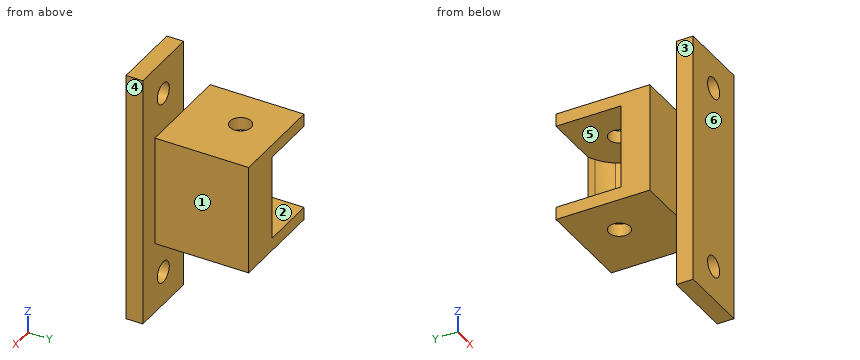
from build123d import *

# Parameters (mm, degrees)
BOSS_EXTRUDE1_DEPTH = 29.21
SKETCH2_R           = 3.175
BOSS_EXTRUDE2_DEPTH = 3.81
BOSS_EXTRUDE4_START = 3.81
SKETCH3_W           = 29.223613814
SKETCH3_H           = 28.25489527
SKETCH3_R           = 3.175
BOSS_EXTRUDE4_DEPTH = 3.81
SKETCH4_W           = 21.59
SKETCH4_H           = 76.2
SKETCH4_R           = 3.175
BOSS_EXTRUDE5_DEPTH = 5.08


with BuildPart() as part:
    # Sketch1 → Boss-Extrude1 (new body)
    with BuildSketch(Plane.XY):
        with BuildLine():
            Line((497.233946268, 332.485515977), (497.233946268, 323.779975182))
            Line((497.233946268, 323.779975182), (526.457560082, 323.779975182))
            Line((526.457560082, 323.779975182), (526.457560082, 352.034870452))
            Line((526.457560082, 352.034870452), (514.19218435, 352.034870452))
            Line((514.19218435, 352.034870452), (515.97416853, 351.010540676))
            ThreePointArc((515.97416853, 351.010540676), (518.254444166, 349.336379834), (520.107560082, 347.198990562))
            ThreePointArc((520.107560082, 347.198990562), (520.655570716, 333.67086151), (508.689794246, 327.335975182))
            ThreePointArc((508.689794246, 327.335975182), (505.910190066, 327.86159111), (503.31589155, 328.989459324))
            Line((503.31589155, 328.989459324), (497.233946268, 332.485515977))
        make_face()
    extrude(amount=-BOSS_EXTRUDE1_DEPTH)

    # Sketch2 → Boss-Extrude2 (add)
    with BuildSketch(Plane(origin=(0, 0, -25.4), x_dir=(-1, 0, 0), z_dir=(0, 0, -1))):
        with BuildLine():
            Line((-514.19218435, 352.034870452), (-497.233946268, 352.034870452))
            Line((-497.233946268, 352.034870452), (-497.233946268, 332.485515977))
            Line((-497.233946268, 332.485515977), (-503.31589155, 328.989459324))
            ThreePointArc((-503.31589155, 328.989459324), (-520.655570716, 333.67086151), (-515.97416853, 351.010540676))
            Line((-515.97416853, 351.010540676), (-514.19218435, 352.034870452))
        make_face()
        with Locations(Location((-509.64503004, 340, 0), (0, 0, 180))):
            Circle(SKETCH2_R, mode=Mode.SUBTRACT)
    extrude(amount=BOSS_EXTRUDE2_DEPTH)

    # Sketch3 → Boss-Extrude4 (add)
    with BuildSketch(Plane.XY.offset(BOSS_EXTRUDE4_START)):
        with Locations((511.845753175, 337.907422817)):
            Rectangle(SKETCH3_W, SKETCH3_H)
        with Locations((509.64503004, 340)):
            Circle(SKETCH3_R, mode=Mode.SUBTRACT)
    extrude(amount=-BOSS_EXTRUDE4_DEPTH)

    # Sketch4 → Boss-Extrude5 (add)
    with BuildSketch(Plane(origin=(0, 323.779975182, 0), x_dir=(1, 0, 0), z_dir=(0, 1, 0))):
        with Locations((522.012560082, 12.7)):
            Rectangle(SKETCH4_W, SKETCH4_H)
        with Locations(Location((522.012560082, 40.64, 0), (0, 0, 270))):
            Circle(SKETCH4_R, mode=Mode.SUBTRACT)
        with Locations(Location((522.012560082, -15.24, 0), (0, 0, 270))):
            Circle(SKETCH4_R, mode=Mode.SUBTRACT)
    extrude(amount=-BOSS_EXTRUDE5_DEPTH)


solid = part.part
Check sheet for the modelled part. Datum: model origin and axes. Units: mm. Face numbers are marked on the shaded views. A direction names the side the tool comes from. Round coordinates to 2 decimals unless told otherwise and drop trailing zeros. Order: outer loops, then holes, each group sorted by start corner. A loop starts at its lowest first (then second) coordinate and runs counter-clockwise, first axis right, second up.
(1) Cross-section at B-B, the plane y = 340. Enter the section's corners in (x, z).
(2) Draft check along X on the marked faces 4, 5 and 6. Enter one of: pulls with the +X half, pulls with the -X half, needs draft (parallel to the pull), parting line crosses it, or undercut.
(3) Go/stop test with flat-tipped pins: P1, Ø12.5, axis at x = 505.5, y = 339.5, coming from the +Z side; P2, Ø20, axis at x = 514, y = 339.5, coming from the -Z side; P3, Ø4, axis at y = 334.5, z = -21.5, coming from the +X side. Record where each tip stops, or that it passes through.
(4) Scan lines: probe 1 along Z at (x, y) = (505.5, 330); probe 2 along X at (y, z) = (321.55, -40.64); probe 3 along X at (y, z) = (340, -27.75). Record each from-to range of solid material in increasing order.
(5) Cross-section at D-D, the plane y = 349. Enter the section's corners in (x, z), and give its area (3 significant figures).
(6) Access from +Z, -Z, +X, -X, +Y, -Y to the whole of each face (thin tool, end or side, straight path). Record for the marked faces 1, 2 and 3.
(7) Cross-section at A-A, the plane z = -40.64. Enter the section's corners in (x, y).
Check sheet entries:
1. outline: (497.23, -29.21) - (506.47, -29.21) - (506.47, -25.4) - (497.23, -25.4) - close; (497.23, 0) - (506.47, 0) - (506.47, 3.81) - (497.23, 3.81) - close; (512.82, -29.21) - (526.46, -29.21) - (526.46, 3.81) - (512.82, 3.81) - (512.82, 0) - (522.35, 0) - (522.35, -25.4) - (512.82, -25.4) - close
2. face 4: pulls with the +X half
2. face 5: undercut
2. face 6: needs draft
3. P1: stops at z = 3.81
3. P2: stops at z = -29.21
3. P3: stops at x = 526.46
4. probe 1: z = -29.21 to -25.4, 0 to 3.81
4. probe 2: x = 511.22 to 518.84, 525.19 to 532.81
4. probe 3: x = 497.23 to 506.47, 512.82 to 526.46
5. outline: (497.23, -29.21) - (526.46, -29.21) - (526.46, 3.81) - (497.23, 3.81) - (497.23, 0) - (518.61, 0) - (518.61, -25.4) - (497.23, -25.4) - close
5. area: 422 mm2
6. face 1: +Z, -Z, +X, +Y
6. face 2: none
6. face 3: +Z, -Z, -X, -Y
7. outline: (511.22, 318.7) - (518.84, 318.7) - (518.84, 323.78) - (511.22, 323.78) - close; (525.19, 318.7) - (532.81, 318.7) - (532.81, 323.78) - (525.19, 323.78) - close
